from build123d import *

# Parameters (mm, degrees)
SKETCH1_W           = 133
SKETCH1_H           = 95
BOSS_EXTRUDE1_DEPTH = 50
CUT_EXTRUDE1_START  = -2
CUT_EXTRUDE1_DEPTH  = 129
SKETCH3_R           = 42.5
CUT_EXTRUDE2_DEPTH  = 10
FILLET1_R           = 2.5
SKETCH4_W           = 50
SKETCH4_H           = 45
BOSS_EXTRUDE2_DEPTH = 6
SKETCH5_R           = 2.525
CUT_EXTRUDE3_DEPTH  = 4


with BuildPart() as part:
    # Sketch1 → Boss-Extrude1 (new body)
    with BuildSketch(Plane(origin=(0, 0, 0), x_dir=(1, 0, 0), z_dir=(0, 1, 0))):
        with Locations((66.5, 47.5)):
            Rectangle(SKETCH1_W, SKETCH1_H)
    extrude(amount=BOSS_EXTRUDE1_DEPTH)

    # Sketch2 → Cut-Extrude1 (cut)
    with BuildSketch(Plane.ZY.offset(CUT_EXTRUDE1_START)):
        with BuildLine():
            Line((-94, 0), (-1, 0))
            ThreePointArc((-1, 0), (-47.5, 46.5), (-94, 0))
        make_face()
    extrude(amount=-CUT_EXTRUDE1_DEPTH, mode=Mode.SUBTRACT)

    # Sketch3 → Cut-Extrude2 (cut)
    with BuildSketch(Plane.ZY):
        with Locations((-47.5, 0)):
            Circle(SKETCH3_R)
    extrude(amount=-CUT_EXTRUDE2_DEPTH, mode=Mode.SUBTRACT)

    # Fillet1
    # the kernel refuses this fillet: 2.5 mm, written as the material it takes off along each edge
    with BuildSketch(Plane(origin=(130.5, 47.5, -92.5), x_dir=(0, 1, 0), z_dir=(1, 0, 0))) as fillet1_piece_1_section:
        Polygon((0, 0), (FILLET1_R * 1.02, 0), (FILLET1_R * 1.02, -FILLET1_R * 1.02), (0, -FILLET1_R * 1.02), align=None)
    fillet1_piece_1 = extrude(amount=FILLET1_R * 1.02, mode=Mode.PRIVATE)
    fillet1_piece_1 = fillet1_piece_1 - Plane(origin=(130.5, 47.5, -92.5), x_dir=(0, -0.7071067811865475, 0.7071067811865475), z_dir=(1, 0, 0)) * Sphere(FILLET1_R, mode=Mode.PRIVATE)
    add(fillet1_piece_1, mode=Mode.SUBTRACT)
    with BuildSketch(Plane(origin=(2.5, 47.5, -92.5), x_dir=(0, 1, 0), z_dir=(-1, 0, 0))) as fillet1_piece_2_section:
        Polygon((0, 0), (FILLET1_R * 1.02, 0), (FILLET1_R * 1.02, FILLET1_R * 1.02), (0, FILLET1_R * 1.02), align=None)
    fillet1_piece_2 = extrude(amount=FILLET1_R * 1.02, mode=Mode.PRIVATE)
    fillet1_piece_2 = fillet1_piece_2 - Plane(origin=(2.5, 47.5, -92.5), x_dir=(0, -0.7071067811865475, 0.7071067811865475), z_dir=(-1, 0, 0)) * Sphere(FILLET1_R, mode=Mode.PRIVATE)
    add(fillet1_piece_2, mode=Mode.SUBTRACT)
    with BuildSketch(Plane(origin=(130.5, 47.5, -2.5), x_dir=(1, 0, 0), z_dir=(0, 0, 1))) as fillet1_piece_3_section:
        Polygon((0, 0), (FILLET1_R * 1.02, 0), (FILLET1_R * 1.02, FILLET1_R * 1.02), (0, FILLET1_R * 1.02), align=None)
    fillet1_piece_3 = extrude(amount=FILLET1_R * 1.02, mode=Mode.PRIVATE)
    fillet1_piece_3 = fillet1_piece_3 - Plane(origin=(130.5, 47.5, -2.5), x_dir=(-0.7071067811865475, -0.7071067811865475, 0), z_dir=(0, 0, 1)) * Sphere(FILLET1_R, mode=Mode.PRIVATE)
    add(fillet1_piece_3, mode=Mode.SUBTRACT)
    with BuildSketch(Plane(origin=(2.5, 47.5, -2.5), x_dir=(-1, 0, 0), z_dir=(0, 0, 1))) as fillet1_piece_4_section:
        Polygon((0, 0), (FILLET1_R * 1.02, 0), (FILLET1_R * 1.02, -FILLET1_R * 1.02), (0, -FILLET1_R * 1.02), align=None)
    fillet1_piece_4 = extrude(amount=FILLET1_R * 1.02, mode=Mode.PRIVATE)
    fillet1_piece_4 = fillet1_piece_4 - Plane(origin=(2.5, 47.5, -2.5), x_dir=(0.7071067811865475, -0.7071067811865475, 0), z_dir=(0, 0, 1)) * Sphere(FILLET1_R, mode=Mode.PRIVATE)
    add(fillet1_piece_4, mode=Mode.SUBTRACT)
    with BuildSketch(Plane(origin=(130.5, 50, -95), x_dir=(0, 0, 1), z_dir=(-1, 0, 0))) as fillet1_piece_5:
        with BuildLine():
            CenterArc((FILLET1_R, -FILLET1_R), FILLET1_R, 90, 90)
            Line((0, -FILLET1_R), (0, 0))
            Line((0, 0), (FILLET1_R, 0))
        make_face()
    extrude(amount=128, mode=Mode.SUBTRACT)
    with BuildSketch(Plane(origin=(133, 50, -2.5), x_dir=(0, -1, 0), z_dir=(0, 0, -1)), Plane(origin=(0, 50, -92.5), x_dir=(0, -1, 0), z_dir=(0, 0, 1))) as fillet1_piece_6:
        with BuildLine():
            CenterArc((FILLET1_R, FILLET1_R), FILLET1_R, 180, 90)
            Line((0, FILLET1_R), (0, 0))
            Line((0, 0), (FILLET1_R, 0))
        make_face()
    extrude(amount=90, mode=Mode.SUBTRACT)
    with BuildSketch(Plane(origin=(2.5, 50, 0), x_dir=(0, -1, 0), z_dir=(1, 0, 0))) as fillet1_piece_7:
        with BuildLine():
            CenterArc((FILLET1_R, FILLET1_R), FILLET1_R, 180, 90)
            Line((0, FILLET1_R), (0, 0))
            Line((0, 0), (FILLET1_R, 0))
        make_face()
    extrude(amount=128, mode=Mode.SUBTRACT)
    with BuildSketch(Plane(origin=(133, -6.25, 0), x_dir=(-1, 0, 0), z_dir=(0, 1, 0)), Plane(origin=(133, -6.25, -95), x_dir=(0, 0, 1), z_dir=(0, 1, 0))) as fillet1_piece_8:
        with BuildLine():
            CenterArc((FILLET1_R, -FILLET1_R), FILLET1_R, 90, 90)
            Line((0, -FILLET1_R), (0, 0))
            Line((0, 0), (FILLET1_R, 0))
        make_face()
    extrude(amount=53.75, mode=Mode.SUBTRACT)
    with BuildSketch(Plane(origin=(133, 0, 6.25), x_dir=(0, 1, 0), z_dir=(0, 0, -1))) as fillet1_piece_9:
        with BuildLine():
            CenterArc((FILLET1_R, -FILLET1_R), FILLET1_R, 90, 90)
            Line((0, -FILLET1_R), (0, 0))
            Line((0, 0), (FILLET1_R, 0))
        make_face()
    extrude(amount=107.5, mode=Mode.SUBTRACT)
    with BuildSketch(Plane(origin=(0, -6.25, -95), x_dir=(0, 0, 1), z_dir=(0, 1, 0)), Plane(origin=(0, -6.25, 0), x_dir=(1, 0, 0), z_dir=(0, 1, 0))) as fillet1_piece_10:
        with BuildLine():
            CenterArc((FILLET1_R, FILLET1_R), FILLET1_R, 180, 90)
            Line((0, FILLET1_R), (0, 0))
            Line((0, 0), (FILLET1_R, 0))
        make_face()
    extrude(amount=53.75, mode=Mode.SUBTRACT)
    with BuildSketch(Plane(origin=(0, 0, -11.25), x_dir=(0, 1, 0), z_dir=(0, 0, 1)), Plane(origin=(0, 0, -101.25), x_dir=(0, 1, 0), z_dir=(0, 0, 1))) as fillet1_piece_11:
        with BuildLine():
            CenterArc((FILLET1_R, -FILLET1_R), FILLET1_R, 90, 90)
            Line((0, -FILLET1_R), (0, 0))
            Line((0, 0), (FILLET1_R, 0))
        make_face()
    extrude(amount=17.5, mode=Mode.SUBTRACT)
    with BuildSketch(Plane(origin=(0, 0, -47.5), x_dir=(0, -0.14381889116089108, 0.9896040251258338), z_dir=(0, -0.9896040251258338, -0.14381889116089108))) as fillet1_piece_12:
        with BuildLine():
            CenterArc((44.949489743, -2.5), FILLET1_R, 90, 78.463040967)
            Line((42.5, -2), (42.5, 0))
            Line((42.5, 0), (44.949489743, 0))
        make_face()
    revolve(axis=Axis((0, 0, -47.5), (-1, 0, 0)), revolution_arc=196.537779553, mode=Mode.SUBTRACT)

    # Sketch4 → Boss-Extrude2 (add)
    with BuildSketch(Plane(origin=(0, 50, 0), x_dir=(1, 0, 0), z_dir=(0, 1, 0))):
        with Locations((66.5, 47.5)):
            Rectangle(SKETCH4_W, SKETCH4_H)
    extrude(amount=BOSS_EXTRUDE2_DEPTH)

    # Sketch5 → Cut-Extrude3 (cut)
    with BuildSketch(Plane(origin=(0, 56, 0), x_dir=(1, 0, 0), z_dir=(0, 1, 0))):
        with Locations(Location((47.5, 63.5, 0), (0, 0, 270))):
            Circle(SKETCH5_R)
        with Locations(Location((85.5, 63.5, 0), (0, 0, 270))):
            Circle(SKETCH5_R)
        with Locations(Location((85.5, 31.5, 0), (0, 0, 270))):
            Circle(SKETCH5_R)
        with Locations(Location((47.5, 31.5, 0), (0, 0, 270))):
            Circle(SKETCH5_R)
    extrude(amount=-CUT_EXTRUDE3_DEPTH, mode=Mode.SUBTRACT)


solid = part.part
Here's how the part is built. I have some questions about the finished solid (model axes, mm). A direction names the side the tool comes from. Round coordinates to 2 decimals unless told otherwise and drop trailing zeros. Loops run counter-clockwise (first coordinate to the right, second up) from the corner with the lowest first, then second, coordinate; pieces in that order, holes last.
1. If we section it at C-C on z = -47.5: Write out the boundary of the cut face in (x, y), plus the area to 3 significant figures.
Answer list:
outline: (0, 44.95) arc R2.5 ccw to (2, 42.5) - (2, 46.5) - (131, 46.5) - (131, 0.05) arc R2.5 ccw to (133, 2.5) - (133, 47.5) arc R2.5 ccw to (130.5, 50) - (91.5, 50) - (91.5, 56) - (41.5, 56) - (41.5, 50) - (2.5, 50) arc R2.5 ccw to (0, 47.5) - close
area: 861 mm2
2. If we section it at B-B on x = 85.5: Write out the boundary of the cut face in (y, z) (3 decimals), plus the area to 3 significant figures.
Answer list:
outline: (0, -95) - (47.5, -95) arc R2.5 ccw to (50, -92.5) - (50, -70) - (56, -70) - (56, -66.025) - (52, -66.025) - (52, -60.975) - (56, -60.975) - (56, -34.025) - (52, -34.025) - (52, -28.975) - (56, -28.975) - (56, -25) - (50, -25) - (50, -2.5) arc R2.5 ccw to (47.5, 0) - (0, 0) - (0, -1) arc R46.5 cw to (0, -94) - close
area: 1,580 mm2
3. If we section it at D-D on x = 15.5: Write out the boundary of the cut face in (y, z), plus the area to 3 significant figures.
Answer list:
outline: (0, -95) - (47.5, -95) arc R2.5 ccw to (50, -92.5) - (50, -2.5) arc R2.5 ccw to (47.5, 0) - (0, 0) - (0, -1) arc R46.5 cw to (0, -94) - close
area: 1,350 mm2
4. For P1, Ø3, axis at x = 47.5, z = -63.5, coming from the -Y side; P2, Ø1.8, axis at x = 69.5, y = 52, coming from the +Z side; P3, Ø6, axis at x = 87, z = -19, coming from the -Y side, each with a flat end and sliding along its axis, tell me the tip position at first contact or that it passes through.
Answer list:
P1: stops at y = 43.08
P2: stops at z = -25
P3: stops at y = 34.21
5. If I drill on line 1 along X through (y, z) = (55.2, -31.5) (3 decimals); line 2 along Z through (x, y) = (47, 53) (3 decimals); line 3 along X through (y, z) = (16, -26), over which ranges is the centre line in solid material (lowest first)?
Answer list:
line 1: x = 41.5 to 44.975, 50.025 to 82.975, 88.025 to 91.5
line 2: z = -70 to -65.975, -61.025 to -33.975, -29.025 to -25
line 3: x = 131 to 133
6. Which directions (+Z, -Z, +X, -X, +Y, -Y) give clear straight access to the entire face, cutting with the end or side of a thin tool? Please do faces 1 (the face through (48, 52, -64)), 2 (the face through (66, 53, -25)), 3 (the face through (41.5, 53, -47)), 4 (the face through (2, 42, -55)).
Answer list:
face 1: +Y
face 2: +Z, +X, -X, +Y
face 3: +Z, -Z, -X, +Y
face 4: -Y
7. We'd pull the mould along Z, two halves only. Please class faces 5 (the face through (66, 56, -48)), 6 (the face through (65.6, 46.49, -46.48)), 7 (the face through (66, 23, 0)): +Z half, -Z half, draft (parallel to the pull), parting line (faces both ways), or undercut.
Answer list:
face 5: draft
face 6: undercut
face 7: +Z half
8. If we section it at A-A on y = 53.5: Write out the boundary of the cut face in (x, z) (3 decimals), plus the area to 3 significant figures.
Answer list:
outline: (41.5, -70) - (91.5, -70) - (91.5, -25) - (41.5, -25) - close; hole circle Ø5.05 at (47.5, -63.5); hole circle Ø5.05 at (47.5, -31.5); hole circle Ø5.05 at (85.5, -63.5); hole circle Ø5.05 at (85.5, -31.5)
area: 2,170 mm2
